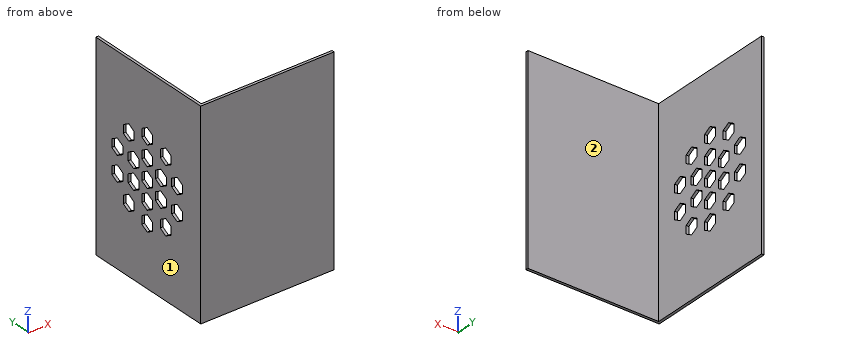
```python
from build123d import *

# Parameters (mm, degrees)
BOSS_EXTRUDE1_DEPTH = 150
FILL_PATTERN1_DEPTH = 2


# Read off the part's stored shape, not the designer's step: Fill Pattern1
with BuildPart() as part:
    # Sketch1 → Boss-Extrude1 (new body)
    with BuildSketch(Plane.XY):
        Polygon((0, 0), (100, 0), (100, 2), (2, 2), (2, 100), (0, 100), align=None)
    extrude(amount=BOSS_EXTRUDE1_DEPTH)

    # Fill Pattern1 outline → Fill Pattern1 (cut)
    with BuildSketch(Plane.YZ):
        Polygon((51, 81), (45.803847577, 78), (45.803847577, 72), (51, 69), (56.196152423, 72), (56.196152423, 78), align=None)
        Polygon((63.990381057, 88.5), (58.794228634, 85.5), (58.794228634, 79.5), (63.990381057, 76.5), (69.186533479, 79.5), (69.186533479, 85.5), align=None)
        Polygon((38.009618943, 73.5), (32.813466521, 70.5), (32.813466521, 64.5), (38.009618943, 61.5), (43.205771366, 64.5), (43.205771366, 70.5), align=None)
        Polygon((45.803847577, 63), (45.803847577, 57), (51, 54), (56.196152423, 57), (56.196152423, 63), (51, 66), align=None)
        Polygon((45.803847577, 108), (45.803847577, 102), (51, 99), (56.196152423, 102), (56.196152423, 108), (51, 111), align=None)
        Polygon((45.803847577, 93), (45.803847577, 87), (51, 84), (56.196152423, 87), (56.196152423, 93), (51, 96), align=None)
        Polygon((45.803847577, 48), (45.803847577, 42), (51, 39), (56.196152423, 42), (56.196152423, 48), (51, 51), align=None)
        Polygon((58.794228634, 64.5), (63.990381057, 61.5), (69.186533479, 64.5), (69.186533479, 70.5), (63.990381057, 73.5), (58.794228634, 70.5), align=None)
        Polygon((32.813466521, 79.5), (38.009618943, 76.5), (43.205771366, 79.5), (43.205771366, 85.5), (38.009618943, 88.5), (32.813466521, 85.5), align=None)
        Polygon((79.531695489, 90.270509831), (74.335543066, 87.270509831), (74.335543066, 81.270509831), (79.531695489, 78.270509831), (84.727847912, 81.270509831), (84.727847912, 87.270509831), align=None)
        Polygon((74.335543066, 68.729490169), (74.335543066, 62.729490169), (79.531695489, 59.729490169), (84.727847912, 62.729490169), (84.727847912, 68.729490169), (79.531695489, 71.729490169), align=None)
        Polygon((68.633557569, 105.270509831), (63.437405146, 102.270509831), (63.437405146, 96.270509831), (68.633557569, 93.270509831), (73.829709991, 96.270509831), (73.829709991, 102.270509831), align=None)
        Polygon((63.437405146, 53.729490169), (63.437405146, 47.729490169), (68.633557569, 44.729490169), (73.829709991, 47.729490169), (73.829709991, 53.729490169), (68.633557569, 56.729490169), align=None)
        Polygon((33.366442431, 105.270509831), (28.170290009, 102.270509831), (28.170290009, 96.270509831), (33.366442431, 93.270509831), (38.562594854, 96.270509831), (38.562594854, 102.270509831), align=None)
        Polygon((28.170290009, 53.729490169), (28.170290009, 47.729490169), (33.366442431, 44.729490169), (38.562594854, 47.729490169), (38.562594854, 53.729490169), (33.366442431, 56.729490169), align=None)
        Polygon((22.468304511, 90.270509831), (17.272152088, 87.270509831), (17.272152088, 81.270509831), (22.468304511, 78.270509831), (27.664456934, 81.270509831), (27.664456934, 87.270509831), align=None)
        Polygon((17.272152088, 68.729490169), (17.272152088, 62.729490169), (22.468304511, 59.729490169), (27.664456934, 62.729490169), (27.664456934, 68.729490169), (22.468304511, 71.729490169), align=None)
    extrude(amount=FILL_PATTERN1_DEPTH, mode=Mode.SUBTRACT)


solid = part.part
```
Model file for the job. Use its own axes, mm. Face numbers are marked on the shaded views. A direction names the side the tool comes from. Give positions to 0.01 mm unless a question says otherwise; leave off trailing zeros. Order: outer loops, then holes, each group sorted by start corner. A loop starts at its lowest first (then second) coordinate and runs counter-clockwise, first axis right, second up.
1) 3-axis set-ups, long thin cutter, end or side, ignore diameter. For the marked faces 1 and 2: which of +Z, -Z, +X, -X, +Y, -Y reach the whole face in a straight line?
2) Pin check, flat tips, straight feed: pin 1 (5 mm diameter, centred on y = 21.5, z = 43, fed in from +X); pin 2 (2 mm diameter, centred on x = 15, z = 122, fed in from +Y). Stop position of each tip, or through.
3) Saw through at C-C, the plane x = 26.5. Write the cut outline in (y, z), then the cut area to 3 significant figures.
4) Saw through at B-B, the plane z = 29. Write the cut outline in (x, y).
5) Saw through at A-A, the plane y = 66.5. Write the cut outline in (x, z), then the cut area to 3 significant figures.
6) Wall check: probe 1 along Y at (x, z) = (52, 130.5). Give the ranges that are in metal, low to high.
Computed:
1. face 1: +Z, -Z, -X, +Y, -Y
1. face 2: +Z, -Z, +X, +Y
2. pin 1: stops at x = 2
2. pin 2: stops at y = 2
3. outline: (0, 0) - (2, 0) - (2, 150) - (0, 150) - close
3. area: 300 mm2
4. outline: (0, 0) - (100, 0) - (100, 2) - (2, 2) - (2, 100) - (0, 100) - close
5. outline: (0, 0) - (2, 0) - (2, 45.96) - (0, 45.96) - close; (0, 55.5) - (2, 55.5) - (2, 62.95) - (0, 62.95) - close; (0, 72.05) - (2, 72.05) - (2, 77.95) - (0, 77.95) - close; (0, 87.05) - (2, 87.05) - (2, 94.5) - (0, 94.5) - close; (0, 104.04) - (2, 104.04) - (2, 150) - (0, 150) - close
5. area: 225 mm2
6. probe 1: y = 0 to 2
